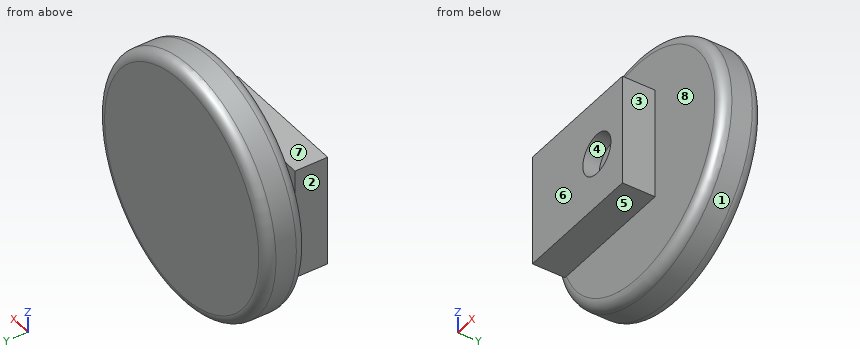
```python
from build123d import *

# Parameters (mm, degrees)
F0_R     = 30
F1_DEPTH = 10
F2_R     = 2.5
F3_R     = 2.5
F4_R     = 5
F5_DEPTH = 6
F6_W     = 32.103093341
F6_H     = 27.4639837444
F6_R     = 5
F7_DEPTH = 4


with BuildPart() as f1:
    # F0 (on Front) → F1 (new body)
    with BuildSketch(Plane.XZ):
        Circle(F0_R)
    extrude(amount=F1_DEPTH)

    # F2
    f2_edges = [f1.edges().sort_by_distance(p)[0] for p in [
        (-30, -10, 0),
    ]]
    fillet(f2_edges, radius=F2_R)

    # F3
    f3_edges = [f1.edges().sort_by_distance(p)[0] for p in [
        (-30, 0, 0),
        (-27.5, -10, 0),
    ]]
    fillet(f3_edges, radius=F3_R)

    # F4 (on face) → F5 (join)
    with BuildSketch(Plane.XZ.offset(10)):
        Circle(F4_R)
    extrude(amount=F5_DEPTH)

    # F6 (on face) → F7 (join, symmetric)
    with BuildSketch(Plane.XZ.offset(16)):
        with Locations((-6.9443220273, 0.3692498431)):
            Rectangle(F6_W, F6_H)
        Circle(F6_R, mode=Mode.SUBTRACT)
    extrude(amount=F7_DEPTH, both=True)


solid = f1.part
```
Build history of the part. All positions in model axes, mm. Face numbers are marked on the shaded views. A direction names the side the tool comes from. Coordinates: 2 decimals unless noted, no trailing zeros. Write each loop counter-clockwise with the first axis right and the second up, starting at its lowest first coordinate (ties: lowest second). Pieces come first, ordered by that corner, then holes.
1. Drop flat-ended pins along their axis: pin 1 (3 mm diameter, centred on y = -14, z = -3.5, fed in from +X); pin 2 (8 mm diameter, centred on x = -19, y = -15.5, fed in from -Z); pin 3 (4 mm diameter, centred on x = -3.5, y = -17.5, fed in from +Z). Give the stop position or say it passes through.
Answer block:
pin 1: stops at x = 9.11
pin 2: stops at z = -13.36
pin 3: stops at z = 14.1
2. Band-saw the part on B-B, the plane x = 0. Give the cut face in (y, z), and give its area (3 significant figures).
Answer block:
outline: (-20, -13.36) - (-12, -13.36) - (-12, -5) - (-10, -5) - (-10, -27.5) arc R2.5 ccw to (-7.5, -30) - (-2.5, -30) arc R2.5 ccw to (0, -27.5) - (0, 27.5) arc R2.5 ccw to (-2.5, 30) - (-7.5, 30) arc R2.5 ccw to (-10, 27.5) - (-10, 5) - (-12, 5) - (-12, 14.1) - (-20, 14.1) - (-20, 5) - (-16, 5) - (-16, -5) - (-20, -5) - close
area: 794 mm2
3. Drill centre lines: probe 1 along Z at (x, y) = (0, -18.7); probe 2 along Y at (x, z) = (-15, 8.5); probe 3 along Y at (x, z) = (15.5, 12.5). Where is each one in solid material? Low to high.
Answer block:
probe 1: z = -13.36 to -5, 5 to 14.1
probe 2: y = -20 to -12, -10 to 0
probe 3: y = -10 to 0
4. 3-axis set-ups, long thin cutter, end or side, ignore diameter. For the marked faces 1, 2, 3, 4 and 5: which of +Z, -Z, +X, -X, +Y, -Y reach the whole face in a straight line?
Answer block:
face 1: +Y, -Y
face 2: +Z, -Z, -X, -Y
face 3: +Z, -Z, +X, -Y
face 4: -Y
face 5: -Z, +X, -X, -Y
5. Pull direction Y, two halves, no side cores. Call the marked faces 6, 7 and 8: released by +Y, released by -Y, zero draft, split by the parting line, or undercut.
Answer block:
face 6: released by -Y
face 7: zero draft
face 8: undercut
6. Band-saw the part on C-C, the plane y = -4.25. Give the cut face in (x, z).
Answer block:
outline: circle Ø60 at (0, 0)
7. Band-saw the part on A-A, the plane z = 0. Give the cut face in (x, y).
Answer block:
outline: (-30, -7.5) arc R2.5 ccw to (-27.5, -10) - (-5, -10) - (-5, -12) - (-23, -12) - (-23, -20) - (-5, -20) - (-5, -16) - (5, -16) - (5, -20) - (9.11, -20) - (9.11, -12) - (5, -12) - (5, -10) - (27.5, -10) arc R2.5 ccw to (30, -7.5) - (30, -2.5) arc R2.5 ccw to (27.5, 0) - (-27.5, 0) arc R2.5 ccw to (-30, -2.5) - close
